Check sheet for the modelled part. Datum: model origin and axes. Units: mm. A direction names the side the tool comes from. Round coordinates to 2 decimals unless told otherwise and drop trailing zeros. Order: outer loops, then holes, each group sorted by start corner. A loop starts at its lowest first (then second) coordinate and runs counter-clockwise, first axis right, second up.
(1) Sectioned sample at B-B, the plane x = 0. Enter the section's corners in (y, z).
(2) Sectioned sample at D-D, the plane z = -5.5. Enter the section's corners in (x, y), and give its area (3 significant figures).
(3) Sectioned sample at C-C, the plane z = -3.5. Enter the section's corners in (x, y) (1 decimal), and give its area (3 significant figures).
(4) Tool access check on faces 4 (the flat face through (1, -5, -3.969)), 5 (the flat face through (1, 0, -6.35)). Record the directions out of +Z, -Z, +X, -X, +Y, -Y that give a thin tool (end or side, any length) a straight path to the whole face; none if there is none.
(5) Depth check by flat-ended pin: pin 1 (1 mm diameter, centred on y = -3.5, z = -1.5, fed in from -X); pin 2 (5.5 mm diameter, centred on x = 2, y = -1, fed in from +Z); pin 3 (1 mm diameter, centred on y = -2, z = -5, fed in from +X); pin 4 (0.5 mm diameter, centred on x = 0, y = 0, fed in from -Z). Enter the tip coordinate at first touch or a pass-through.
(6) Mould release check, pull along Y, two halves, no side actions. Record for faces 1 (the cylindrical face through (-4.724, 3.622, -5.146)), 2 (the flat face through (0, 0, -5.953)), 3 (the flat face through (0, 0, 0)): released by +Y, released by -Y, zero draft, split by the parting line, or undercut.
(7) Sectioned sample at A-A, the plane y = 0. Enter the section's corners in (x, z), and give its area (3 significant figures).
(8) Thickness scan on probe 1 along Z at (x, y) = (-1.75, 4.5); probe 2 along Y at (x, z) = (0, -1.25); probe 3 along X at (y, z) = (4, -0.75). Record the ranges inside material, lowest first.
```python
from build123d import *

# Parameters (mm, degrees)
FILLET1_R          = 0.20483871
SKETCH2_W          = 1.5875
SKETCH2_H          = 9.525
CUT_EXTRUDE1_DEPTH = 0.396875
CHAMFER1_SIZE      = 0.79375
CHAMFER1_SIZE_2    = 1.374815329


with BuildPart() as part:
    # Sketch1 → Revolve1 (revolve)
    with BuildSketch(Plane(origin=(0, 0, 0), x_dir=(1, 0, 0), z_dir=(0, 1, 0))):
        Polygon((0, 6.35), (5.953125, 6.35), (5.953125, 3.96875), (4.7625, 3.96875), (4.7625, 0.898025612), (3.864474388, 0), (0, 0), align=None)
    revolve(axis=Axis((0, 0, 0), (0, 0, -1)))

    # Fillet1
    fillet1_edges = [part.edges().sort_by_distance(p)[0] for p in [
        (-5.953125, 0, -3.96875),
        (-5.953125, 0, -6.35),
    ]]
    fillet(fillet1_edges, radius=FILLET1_R)

    # Sketch2 → Cut-Extrude1 (cut)
    with BuildSketch(Plane(origin=(0, 0, -6.35), x_dir=(-1, 0, 0), z_dir=(0, 0, -1))):
        Rectangle(SKETCH2_W, SKETCH2_H)
    extrude(amount=-CUT_EXTRUDE1_DEPTH, mode=Mode.SUBTRACT)

    # Chamfer1
    # the kernel refuses this chamfer: 1.374815329, 0.79375 mm, written as the material it adds along each edge
    with BuildSketch(Plane(origin=(-0.79375, -4.7625, -5.953125), x_dir=(0, -0.057893862402671005, -0.9983227437537926), z_dir=(1, 0, 0))) as chamfer1_piece_1_section:
        Polygon((CHAMFER1_SIZE * 0.998322743754, CHAMFER1_SIZE * 0.0578938624027), (-CHAMFER1_SIZE_2 * 0.0578938623819, CHAMFER1_SIZE_2 * 0.998322743396), (0, 0), align=None)
    chamfer1_piece_1 = extrude(amount=1.5875, mode=Mode.PRIVATE)
    chamfer1_piece_1 = split(chamfer1_piece_1, bisect_by=Plane(origin=(0, -4.227849594, -6.35), z_dir=(0, 0, 1)), keep=Keep.TOP, mode=Mode.PRIVATE)
    add(chamfer1_piece_1)
    with BuildSketch(Plane(origin=(0.79375, 4.7625, -5.953125), x_dir=(0, 0.057893862402671005, -0.9983227437537926), z_dir=(-1, 0, 0))) as chamfer1_piece_2_section:
        Polygon((CHAMFER1_SIZE * 0.998322743754, CHAMFER1_SIZE * 0.0578938624027), (-CHAMFER1_SIZE_2 * 0.0578938623819, CHAMFER1_SIZE_2 * 0.998322743396), (0, 0), align=None)
    chamfer1_piece_2 = extrude(amount=1.5875, mode=Mode.PRIVATE)
    chamfer1_piece_2 = split(chamfer1_piece_2, bisect_by=Plane(origin=(0, 4.227849594, -6.35), z_dir=(0, 0, 1)), keep=Keep.TOP, mode=Mode.PRIVATE)
    add(chamfer1_piece_2)


solid = part.part
```
Derived:
1. outline: (-5.95, -6.15) arc R0.2 ccw to (-5.75, -6.35) - (-4.08, -6.35) - (-3.39, -5.95) - (3.39, -5.95) - (4.08, -6.35) - (5.75, -6.35) arc R0.2 ccw to (5.95, -6.15) - (5.95, -4.17) arc R0.2 ccw to (5.75, -3.97) - (4.76, -3.97) - (4.76, -0.9) - (3.86, 0) - (-3.86, 0) - (-4.76, -0.9) - (-4.76, -3.97) - (-5.75, -3.97) arc R0.2 ccw to (-5.95, -4.17) - close
2. outline: circle Ø11.91 at (0, 0)
2. area: 111 mm2
3. outline: circle Ø9.5 at (0, 0)
3. area: 71.3 mm2
4. face 4: +Z
4. face 5: -Z, +X, -X, +Y, -Y
5. pin 1: stops at x = -3.7
5. pin 2: stops at z = 0
5. pin 3: stops at x = 5.76
5. pin 4: stops at z = -5.95
6. face 1: split by the parting line
6. face 2: undercut
6. face 3: zero draft
7. outline: (-5.95, -6.15) arc R0.2 ccw to (-5.75, -6.35) - (-0.79, -6.35) - (-0.79, -5.95) - (0.79, -5.95) - (0.79, -6.35) - (5.75, -6.35) arc R0.2 ccw to (5.95, -6.15) - (5.95, -4.17) arc R0.2 ccw to (5.75, -3.97) - (4.76, -3.97) - (4.76, -0.9) - (3.86, 0) - (-3.86, 0) - (-4.76, -0.9) - (-4.76, -3.97) - (-5.75, -3.97) arc R0.2 ccw to (-5.95, -4.17) - close
7. area: 64.7 mm2
8. probe 1: z = -6.35 to -3.97
8. probe 2: y = -4.76 to 4.76
8. probe 3: x = -2.3 to 2.3
